from build123d import *

# Parameters (mm, degrees)
SKETCH1_R                                    = 2.4892
BOSS_EXTRUDE1_DEPTH                          = 3.175
FILLET1_R                                    = 4.7625
CSK_FOR_10_FLAT_HEAD_MACHINE_SCREW3_AT_COUNT = 2
CSK_FOR_10_FLAT_HEAD_MACHINE_SCREW3_AT_PITCH = 15.875
CSK_FOR_10_FLAT_HEAD_MACHINE_SCREW3_2_COUNT  = 2
CSK_FOR_10_FLAT_HEAD_MACHINE_SCREW3_2_PITCH  = 34.925


with BuildPart() as part:
    # Sketch1 → Boss-Extrude1 (new body)
    with BuildSketch(Plane.XY):
        Polygon((-33.401, 23.749), (-33.401, -21.209), (41.275, -21.209), (41.275, 0.381), (-17.145, 0.381), (-17.145, 23.749), align=None)
        with Locations((-25.4, -11.049)):
            Circle(SKETCH1_R, mode=Mode.SUBTRACT)
        with Locations((-25.4, 1.651)):
            Circle(SKETCH1_R, mode=Mode.SUBTRACT)
        with Locations((-25.4, 14.351)):
            Circle(SKETCH1_R, mode=Mode.SUBTRACT)
        with Locations((-25.4, -11.049)):
            Circle(SKETCH1_R)
    extrude(amount=BOSS_EXTRUDE1_DEPTH)

    # Fillet1
    fillet1_edges = [part.edges().sort_by_distance(p)[0] for p in [
        (-33.401, 23.749, 1.5875),
        (-17.145, 23.749, 1.5875),
        (-17.145, 0.381, 1.5875),
        (41.275, 0.381, 1.5875),
        (41.275, -21.209, 1.5875),
        (-33.401, -21.209, 1.5875),
    ]]
    fillet(fillet1_edges, radius=FILLET1_R)

    # Sketch7 → CSK for #10 Flat Head Machine Screw3 (revolve, cut)
    with BuildSketch(Plane(origin=(31.75, -11.049, 0), x_dir=(0, 1, 0), z_dir=(1, 0, 0))):
        Polygon((0, 0), (0, 3.175), (2.5527, 3.175), (2.5527, 2.688180894), (4.8895, 0), align=None)
    csk_for_10_flat_head_machine_screw3 = revolve(axis=Axis((31.75, -11.049, -6.35), (0, 0, 1)), mode=Mode.SUBTRACT)

    # CSK for #10 Flat Head Machine Screw3 at: CSK for #10 Flat Head Machine Screw3 ×2
    with Locations(*[(-i * CSK_FOR_10_FLAT_HEAD_MACHINE_SCREW3_AT_PITCH, 0, 0) for i in range(1, CSK_FOR_10_FLAT_HEAD_MACHINE_SCREW3_AT_COUNT)]):
        add(csk_for_10_flat_head_machine_screw3, mode=Mode.SUBTRACT)

    # CSK for _10 Flat Head Machine Screw3 2: CSK for #10 Flat Head Machine Screw3 ×2
    with Locations(*[(-i * CSK_FOR_10_FLAT_HEAD_MACHINE_SCREW3_2_PITCH, 0, 0) for i in range(1, CSK_FOR_10_FLAT_HEAD_MACHINE_SCREW3_2_COUNT)]):
        add(csk_for_10_flat_head_machine_screw3, mode=Mode.SUBTRACT)


solid = part.part
Check sheet for the modelled part. Datum: model origin and axes. Units: mm. A direction names the side the tool comes from. Give positions to 0.01 mm unless a question says otherwise; leave off trailing zeros. Write each loop counter-clockwise with the first axis right and the second up, starting at its lowest first coordinate (ties: lowest second). Pieces come first, ordered by that corner, then holes. Notation, with made-up numbers: (78.5, 1) -> (107.5, 1) arc R6 cw to (107.5, 6) -> close; hole circle Ø1 at (-17.75, 51). An arc over 180 degrees is marked (long way). Write item = value, one per line.
Item 1: Sectioned sample at A-A on x = -25.4. Record the boundary of the cut face in (y, z) (3 decimals), and give its area (3 significant figures).
Output:
outline = (-21.209, 0) -> (-0.838, 0) -> (-0.838, 3.175) -> (-21.209, 3.175) -> close; (4.14, 0) -> (11.862, 0) -> (11.862, 3.175) -> (4.14, 3.175) -> close; (16.84, 0) -> (23.749, 0) -> (23.749, 3.175) -> (16.84, 3.175) -> close
area = 111 mm^2
Item 2: Gauge pin test, flat ends, axial feed: pin 1 (1.5 mm diameter, centred on x = 17.5, y = -9.5, fed in from +Z) (3 decimals); pin 2 (1.6 mm diameter, centred on x = 23.5, z = 1.5, fed in from +Y); pin 3 (4.5 mm diameter, centred on x = -25.4, y = 1.651, fed in from -Z); pin 4 (8 mm diameter, centred on x = 15.875, y = -11.049, fed in from -Z). Record the tip position at first contact, or that the pin passes through.
Output:
pin_1 = 3.175
pin_2 = 0.38
pin_3 = through
pin_4 = 1.02
Item 3: Sectioned sample at C-C on y = 16. Record the boundary of the cut face in (x, z) (3 decimals), and give its area (3 significant figures).
Output:
outline = (-33.401, 0) -> (-27.265, 0) -> (-27.265, 3.175) -> (-33.401, 3.175) -> close; (-23.535, 0) -> (-17.145, 0) -> (-17.145, 3.175) -> (-23.535, 3.175) -> close
area = 39.8 mm^2
Item 4: Scan lines: probe 1 along Y at (x, z) = (31.75, 3.05); probe 2 along X at (y, z) = (-11, 2.8) (3 decimals); probe 3 along X at (y, z) = (-13, 0.75) (3 decimals). Record each from-to range of solid material in increasing order. Write a range as from..to.
Output:
probe_1 = -21.21..-13.6, -8.5..0.38
probe_2 = -33.401..-5.727, -0.623..13.323, 18.427..29.198, 34.302..41.275
probe_3 = -33.401..-6.937, 0.587..12.113, 19.637..27.988, 35.512..41.275
Item 5: Sectioned sample at D-D on z = 2.2. Count the separate pieces of the cut face and the enclosed holes in it, and give its area (3 significant figures).
Output:
separate_pieces = 1
enclosed_holes = 5
area = 1,850 mm^2
Item 6: Tool access check on faces 5 (the flat face through (12, 0.381, 2)), 6 (the flat face through (-33.401, 2, 2)). Record the directions out of +Z, -Z, +X, -X, +Y, -Y that give a thin tool (end or side, any length) a straight path to the whole face; none if there is none.
Output:
face_5 = +Z, -Z, +X, +Y
face_6 = +Z, -Z, -X, +Y, -Y
Item 7: Sectioned sample at B-B on x = 31.75. Record the boundary of the cut face in (y, z) (1 decimal).
Output:
outline = (-21.2, 0) -> (-15.9, 0) -> (-13.6, 2.7) -> (-13.6, 3.2) -> (-21.2, 3.2) -> close; (-8.5, 2.7) -> (-6.2, 0) -> (0.4, 0) -> (0.4, 3.2) -> (-8.5, 3.2) -> close
Item 8: Release check for a two-part mould opening along X. For faces 1 (the conical face through (34.385, -11.634, 2.52)), 2 (the cylindrical face through (-32.04, -19.78, 1.61)), 3 (the flat face through (-5, -8, 3.175)), 4 (the cylindrical face through (-18.503, 22.317, 1.61)) record: +X half, -X half, draft (parallel to the pull), parting line (faces both ways), or undercut.
Output:
face_1 = undercut
face_2 = -X half
face_3 = draft
face_4 = +X half
